Autodesk Inventor part; units mm, degrees
ref_plane "YZ Plane" through (0, 0, 0) normal (1, 0, 0) x (0, 1, 0)
ref_plane "XZ Plane" through (0, 0, 0) normal (0, 1, 0) x (-1, 0, 0)
ref_plane "XY Plane" through (0, 0, 0) normal (0, 0, 1) x (1, 0, 0)
sketch "Sketch1" plane through (0, 0, 0) normal (1, 0, 0) x (0, 1, 0)
  line L0 (-3.195, -4.0211) -> (-3.195, -25.8564)
  line L1 (-3.195, -25.8564) -> (19.03, -25.8564)
  line L2 (19.03, -25.8564) -> (19.03, -0.4564)
  line L3 (19.03, -0.4564) -> (23.7925, -0.4564)
  line L4 (23.7925, -0.4564) -> (23.7925, 0)
  line L5 (19.03, 1.1311) -> (-3.195, 1.1311)
  line L6 (-3.195, 1.1311) -> (-3.195, -4.0211)
  line L7 (19.03, 1.1311) -> (19.03, 7.4811)
  line L8 (19.03, 7.4811) -> (23.7925, 7.4811)
  line L9 (23.7925, 7.4811) -> (23.7925, 0)
  dimension "d1" = 4.7625
  dimension "d2" = 7.9375
  dimension "d3" = 6.35
  dimension "d5" = 26.9875
  dimension "d6" = 22.225
revolve "Revolution1" add sketch "Sketch1" angle 360 about axis through (0, -3.195, -4.0211) along (0, 0, -1)
sketch "Sketch2" plane through (0, -3.195, -25.8564) normal (0, 0, -1) x (-1, 0, 0)
  point P0 (0, 3.195)
sketch "Sketch3" plane through (0, -3.195, -25.8564) normal (0, 0, -1) x (-1, 0, 0)
  point P0 (0, 3.195)
  point P1 (0, 0)
hole "Hole1" at (0, -3.195, -25.8564) direction (0, 0, 1) diameter 4.9784 depth 19.05 tip angle 118 countersink diameter 9.525 countersink angle 82
chamfer "Chamfer1" distance 0.762 angle 45 1 edges at (0, -25.42, 7.4811) measured on face at (-3.9258, 21.7283, 7.4811)
chamfer "Chamfer2" distance 0.762 angle 45 1 edges at (0, -25.42, -25.8564) measured on face at (-2.1528, 12.9477, -25.8564)
fillet "Fillet1" radius 0.7874 1 edges at (0, -30.1825, -0.4564)
properties part number "Loer die 2 center" material "Steel"
Check sheet for the modelled part. Datum: model origin and axes. Units: mm. A direction names the side the tool comes from. Round coordinates to 2 decimals unless told otherwise and drop trailing zeros. Order: outer loops, then holes, each group sorted by start corner. A loop starts at its lowest first (then second) coordinate and runs counter-clockwise, first axis right, second up.
Q1. Set-up check for faces 4 (the face through (12, 17, 7.481)), 5 (the face through (-6.676, 18.004, 3.964)), 6 (the face through (-0.11, -5.68, -14.91)): record each of +Z, -Z, +X, -X, +Y, -Y from which the full face is reachable in a straight line by a thin tool's end or side.
Filled sheet:
face 4: +Z, +X, -X, +Y, -Y
face 5: +Z
face 6: -Z
Q2. Scan lines: L1, parallel to Z at x = -21, y = 1; L2, parallel to Z at x = 1, y = 22; L3, parallel to X at y = -2, z = 5. Record each from-to range of solid material in increasing order.
Filled sheet:
L1: z = -25.86 to 1.13
L2: z = -0.46 to 7.48
L3: x = -26.96 to -22.19, 22.19 to 26.96
Q3. Cross-section at A-A, the plane z = -18.5. Enter the section's corners in (x, y) (3 decimals), plus the area to 3 significant figures.
Filled sheet:
outline: circle Ø44.45 at (0, -3.195); hole circle Ø4.978 at (0, -3.195)
area: 1,530 mm2
Q4. Depth check by flat-ended pin: P1, Ø4.5, axis at x = 0, y = -3.195, coming from the +Z side; P2, Ø8, axis at y = 2.5, z = -7.5, coming from the -X side; P3, Ø5, axis at y = -4, z = -9.5, coming from the +X side (3 decimals). Enter the tip coordinate at first touch or a pass-through.
Filled sheet:
P1: stops at z = 1.13
P2: stops at x = -22.16
P3: stops at x = 22.225
Q5. Draft check along Y on faces 1 (the face through (-6.676, 18.004, -12.603)), 2 (the face through (-0.17, -2.8, -5.57)), 3 (the face through (-19.3, -15, -0.456)). Enter one of: pulls with the +Y half, pulls with the -Y half, needs draft (parallel to the pull), parting line crosses it, or undercut.
Filled sheet:
face 1: parting line crosses it
face 2: undercut
face 3: needs draft
